For this review, use the dimensioned drawing (mm, ordinates from the lowest corner) and the shaded views. Coordinates: 2 decimals unless noted, no trailing zeros. Loops run counter-clockwise (first coordinate to the right, second up) from the corner with the lowest first, then second, coordinate; pieces in that order, holes last. Notation, with made-up numbers: (-20, 0.5) - (3, 0.5) arc R20 cw to (3, 35.5) - close; hole circle Ø10 at (20, 72.5). An arc over 180 degrees is marked (long way). Use a Markdown table: item, result. Add a question column.
1) Add section D-D, the plane x = 67. Give the boundary of the cut face in (y, z).
2) Add section B-B, the plane z = 121. Give the boundary of the cut face in (x, y), and give its area (3 significant figures).
3) Add section C-C, the plane x = 31.5. Give the boundary of the cut face in (y, z).
4) Clearance check with a flat-ended pin moving along its axis: pin 1 (1 mm diameter, centred on x = 19, y = 0.5, fed in from -Z). State where the tip first meets the part, or that it passes through.
5) To check wall thickness, follow L1, parallel to X at y = 0.2, z = 113; L2, parallel to X at y = 0.4, z = 113.5; L3, parallel to Z at x = 28, y = 1. State the ranges of each line that lie inside material, in increasing order. Write a range as [from, to].
6) Add section A-A, the plane y = 1.95. Give the boundary of the cut face in (x, z).
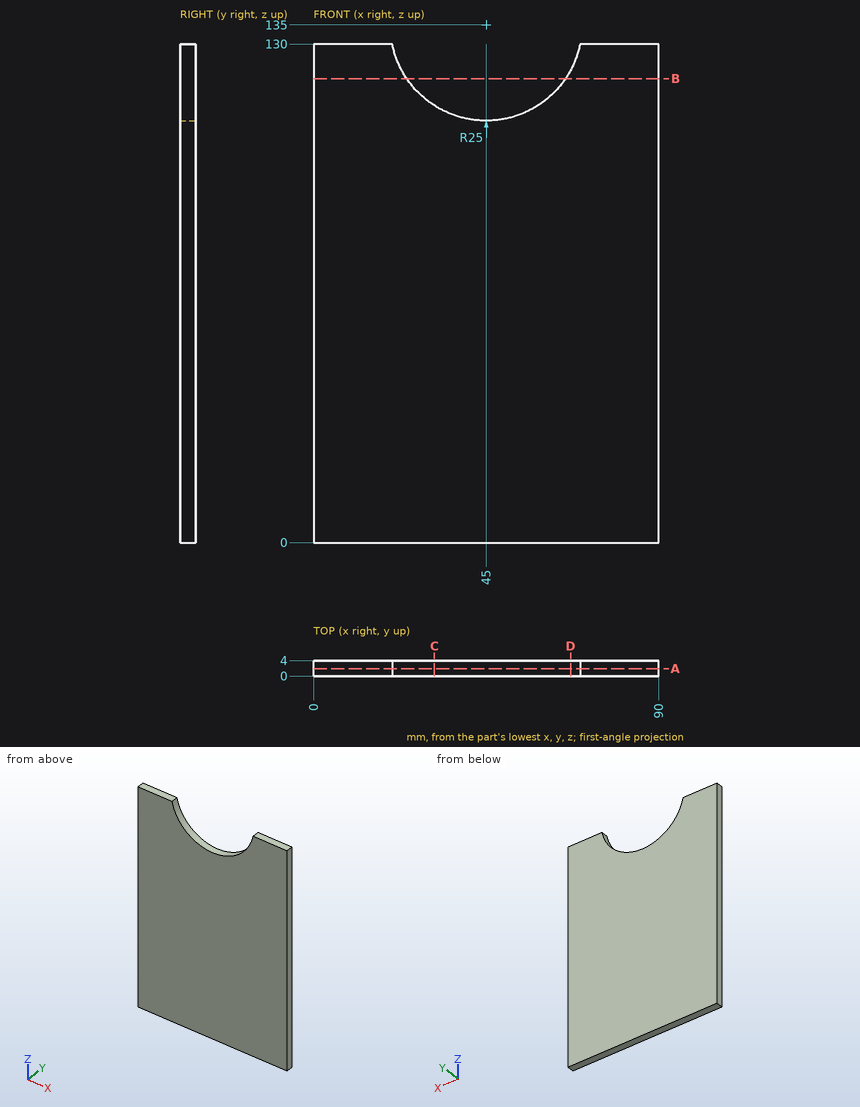
From the geometry:
| question | item | result |
|---|---|---|
| 1 | outline | (0, 0) - (4, 0) - (4, 123.13) - (0, 123.13) - close |
| 2 | outline | (0, 0) - (24.29, 0) - (24.29, 4) - (0, 4) - close; (65.71, 0) - (90, 0) - (90, 4) - (65.71, 4) - close |
| 2 | area | 194 mm^2 |
| 3 | outline | (0, 0) - (4, 0) - (4, 113.96) - (0, 113.96) - close |
| 4 | pin 1 | stops at z = 0 |
| 5 | L1 | x = [0, 33.13], [56.87, 90] |
| 5 | L2 | x = [0, 32.24], [57.76, 90] |
| 5 | L3 | z = [0, 116.67] |
| 6 | outline | (0, 0) - (90, 0) - (90, 130) - (69.49, 130) arc R25 cw to (20.51, 130) - (0, 130) - close |
